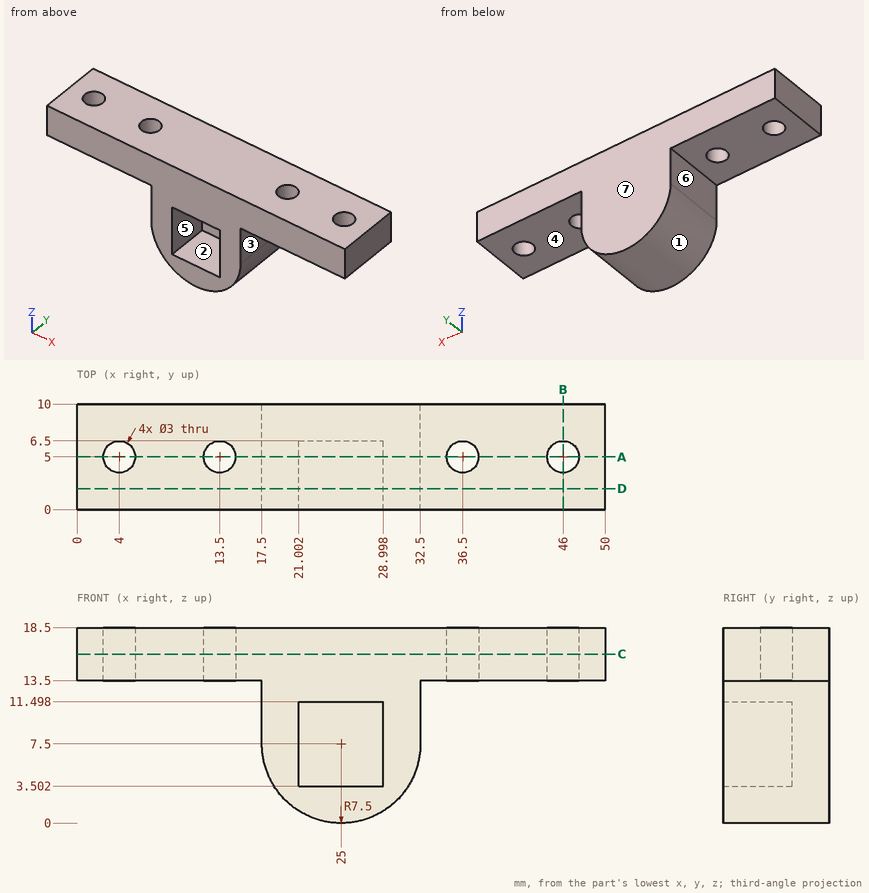
Could you check a few things on this drawing? It's one solid part, dimensions in mm from its lowest x, y, z. A direction names the side the tool comes from. Give positions to 0.01 mm unless a question says otherwise; leave off trailing zeros. Write each loop counter-clockwise with the first axis right and the second up, starting at its lowest first coordinate (ties: lowest second). Pieces come first, ordered by that corner, then holes. Notation, with made-up numbers: (70, 74) -> (89, 74) arc R25 ccw to (89, 106) -> close; hole circle Ø6 at (2.25, 83). An arc over 180 degrees is marked (long way). Answer as CSV lines item,"result". Start each with the question number.
(1) If we section it at B-B, the plane x = 46: Write out the boundary of the cut face in (y, z), and give its area (3 significant figures).
(2) Please list where these lines run through material, in increasing order: line 1 (Y direction, x = 36.5, z = 17.25); line 2 (X direction, y = 3, z = 8); line 3 (Z direction, x = 34, y = 1).
(3) If we section it at C-C, the plane z = 16: Write out the boundary of the cut face in (x, y).
(4) If we mould it in two halves opening along Z, with no side actions, what happens to the marked faces 1, 2 and 3? For each: +Z half, -Z half, draft (parallel to the pull), parting line (faces both ways), or undercut.
(5) I'm going to push flat-ended pins straight in: pin 1 Ø3 at (y, z) = (2.5, 9.5) entering from +X; pin 2 Ø5 at (y, z) = (5, 9.5) entering from -X; pin 3 Ø3.5 at (x, y) = (36.5, 5) entering from -Z. Where does each tip first touch, or does it pass through?
(6) Which directions (+Z, -Z, +X, -X, +Y, -Y) give clear straight access to the entire face, cutting with the end or side of a thin tool? Please do the marked faces 4, 5, 6 and 7.
(7) If we section it at A-A, the plane y = 5: Write out the boundary of the cut face in (x, z).
(8) If we section it at D-D, the plane y = 2: Write out the boundary of the cut face in (x, z).
Answer list:
1,outline,"(0, 13.5) -> (3.5, 13.5) -> (3.5, 18.5) -> (0, 18.5) -> close; (6.5, 13.5) -> (10, 13.5) -> (10, 18.5) -> (6.5, 18.5) -> close"
1,area,"35.0 mm^2"
2,line 1,"0 to 3.5, 6.5 to 10"
2,line 2,"17.5 to 21, 29 to 32.5"
2,line 3,"13.5 to 18.5"
3,outline,"(0, 0) -> (50, 0) -> (50, 10) -> (0, 10) -> close; hole circle Ø3 at (4, 5); hole circle Ø3 at (13.5, 5); hole circle Ø3 at (36.5, 5); hole circle Ø3 at (46, 5)"
4,face 1,"-Z half"
4,face 2,"undercut"
4,face 3,"draft"
5,pin 1,"x = 32.5"
5,pin 2,"x = 17.5"
5,pin 3,"z = 13.5"
6,face 4,"-Z, +X, +Y, -Y"
6,face 5,"-Y"
6,face 6,"-Z, -X, +Y, -Y"
6,face 7,"+Z, -Z, +X, -X, +Y"
7,outline,"(0, 13.5) -> (2.5, 13.5) -> (2.5, 18.5) -> (0, 18.5) -> close; (5.5, 13.5) -> (12, 13.5) -> (12, 18.5) -> (5.5, 18.5) -> close; (15, 13.5) -> (17.5, 13.5) -> (17.5, 7.5) arc R7.5 ccw to (32.5, 7.5) -> (32.5, 13.5) -> (35, 13.5) -> (35, 18.5) -> (15, 18.5) -> close; (38, 13.5) -> (44.5, 13.5) -> (44.5, 18.5) -> (38, 18.5) -> close; (47.5, 13.5) -> (50, 13.5) -> (50, 18.5) -> (47.5, 18.5) -> close; hole (21, 3.5) -> (29, 3.5) -> (29, 11.5) -> (21, 11.5) -> close"
8,outline,"(0, 13.5) -> (17.5, 13.5) -> (17.5, 7.5) arc R7.5 ccw to (32.5, 7.5) -> (32.5, 13.5) -> (50, 13.5) -> (50, 18.5) -> (0, 18.5) -> close; hole (21, 3.5) -> (29, 3.5) -> (29, 11.5) -> (21, 11.5) -> close"
